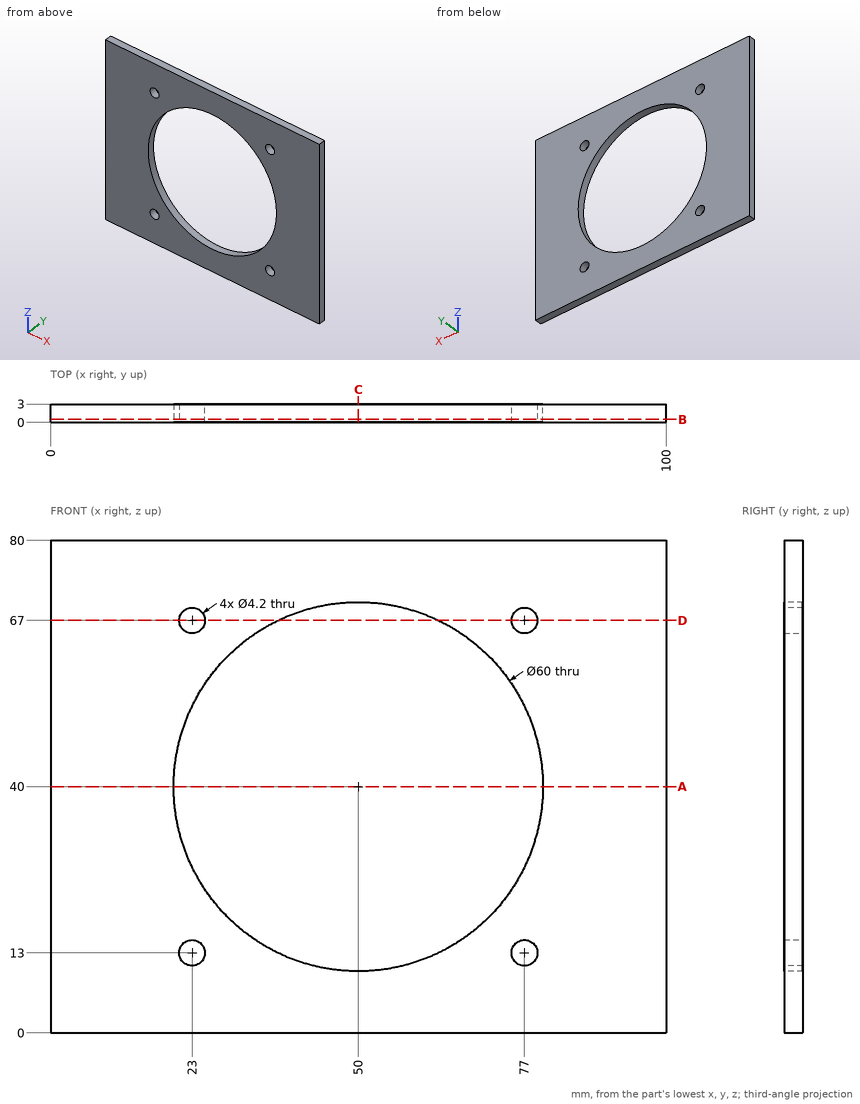
Geometry check sheet. Reference: drawing and pictorial views, mm from the part's lowest x, y, z. Round coordinates to 2 decimals unless told otherwise and drop trailing zeros. Loops run counter-clockwise (first coordinate to the right, second up) from the corner with the lowest first, then second, coordinate; pieces in that order, holes last. Notation, with made-up numbers: (-23.75, 84) - (-1.75, 84) arc R19 cw to (-1.75, 102) - close; hole circle Ø9 at (18, 37.5). An arc over 180 degrees is marked (long way). Use a Markdown table: item, result. Add a question column.
1. Section check C-C, the plane x = 50. Record the boundary of the cut face in (y, z).
2. Section check A-A, the plane z = 40. Record the boundary of the cut face in (x, y), plus the area to 3 significant figures.
3. Section check B-B, the plane y = 0.5. Record the boundary of the cut face in (x, z).
4. Thickness scan on probe 1 along Z at (x, y) = (77, 1.2); probe 2 along Z at (x, y) = (50, 1.3); probe 3 along X at (y, z) = (2.35, 40). Record the ranges inside material, lowest first. Write a range as [from, to].
5. Section check D-D, the plane z = 67. Record the boundary of the cut face in (x, y).
Checks:
| question | item | result |
|---|---|---|
| 1 | outline | (0, 0) - (3, 0) - (3, 10) - (0, 10) - close; (0, 70) - (3, 70) - (3, 80) - (0, 80) - close |
| 2 | outline | (0, 0) - (20, 0) - (20, 3) - (0, 3) - close; (80, 0) - (100, 0) - (100, 3) - (80, 3) - close |
| 2 | area | 120 mm^2 |
| 3 | outline | (0, 0) - (100, 0) - (100, 80) - (0, 80) - close; hole circle Ø60 at (50, 40); hole circle Ø4.2 at (23, 13); hole circle Ø4.2 at (23, 67); hole circle Ø4.2 at (77, 13); hole circle Ø4.2 at (77, 67) |
| 4 | probe 1 | z = [0, 10.9], [15.1, 26.92], [53.08, 64.9], [69.1, 80] |
| 4 | probe 2 | z = [0, 10], [70, 80] |
| 4 | probe 3 | x = [0, 20], [80, 100] |
| 5 | outline | (0, 0) - (20.9, 0) - (20.9, 3) - (0, 3) - close; (25.1, 0) - (36.92, 0) - (36.92, 3) - (25.1, 3) - close; (63.08, 0) - (74.9, 0) - (74.9, 3) - (63.08, 3) - close; (79.1, 0) - (100, 0) - (100, 3) - (79.1, 3) - close |
